Build history of the part. All positions in model axes, mm. Face numbers are marked on the shaded views. A direction names the side the tool comes from. Give positions to 0.01 mm unless a question says otherwise; leave off trailing zeros. Order: outer loops, then holes, each group sorted by start corner. A loop starts at its lowest first (then second) coordinate and runs counter-clockwise, first axis right, second up. Notation, with made-up numbers: (-19, 82.25) - (1, 82.25) arc R20 ccw to (1, 120.25) - close; hole circle Ø6 at (19, 32.25). An arc over 180 degrees is marked (long way). Use a Markdown table: item, result. Add a question column.
(1) Wall check: line 1 (X direction, y = 16.5, z = 31.5); line 2 (Y direction, x = -39, z = 24); line 3 (Z direction, x = -36, y = 10). Give the ranges that are in metal, low to high.
(2) Slice it at B-B (z = 19). Write the cut outline in (x, y), then the cut area to 3 significant figures.
(3) Slice it at A-A (x = -2). Write the cut outline in (y, z), then the cut area to 3 significant figures.
(4) Flat gauge pin, fed straight in: pin 1 (4 mm diameter, centred on x = 17.5, y = 17, fed in from -Z). Where does the tip first touch, or does it go through?
(5) Which spindle directions (+Z, -Z, +X, -X, +Y, -Y) get a long thin tool onto all of the face, cutting with end or side? Do the marked faces 1 and 2. Say none if no direction does.
(6) Slice it at C-C (y = 8). Write the cut outline in (x, z), then the cut area to 3 significant figures.
(7) Mould opens along Y. For the marked faces 3, 4 and 5 say: +Y half, -Y half, draft (parallel to the pull), parting line (faces both ways), or undercut.
from build123d import *

# Parameters (mm, degrees)
SKETCH_W        = 101
SKETCH_H        = 61
PAD_DEPTH       = 42.7
SKETCH001_W     = 91
SKETCH001_H     = 51
POCKET_DEPTH    = 32.7
CHAMFER_SIZE    = 2
CHAMFER001_SIZE = 2
CHAMFER002_SIZE = 2
CHAMFER003_SIZE = 2


with BuildPart() as part:
    # Sketch → Pad (new body)
    with BuildSketch(Plane.XY):
        Rectangle(SKETCH_W, SKETCH_H)
    extrude(amount=PAD_DEPTH)

    # Sketch001 (on Face5 of Pad) → Pocket (cut)
    with BuildSketch(Plane(origin=(0, 0, 0), x_dir=(1, 0, 0), z_dir=(0, 0, -1))):
        Rectangle(SKETCH001_W, SKETCH001_H)
    extrude(amount=-POCKET_DEPTH, mode=Mode.SUBTRACT)

    # Chamfer
    chamfer_edges = [part.edges().sort_by_distance(p)[0] for p in [
        (-50.5, -30.5, 21.35),
    ]]
    chamfer(chamfer_edges, length=CHAMFER_SIZE)

    # Chamfer001
    chamfer001_edges = [part.edges().sort_by_distance(p)[0] for p in [
        (-50.5, 30.5, 21.35),
    ]]
    chamfer(chamfer001_edges, length=CHAMFER001_SIZE)

    # Chamfer002
    chamfer002_edges = [part.edges().sort_by_distance(p)[0] for p in [
        (50.5, 30.5, 21.35),
        (50.5, -30.5, 21.35),
    ]]
    chamfer(chamfer002_edges, length=CHAMFER002_SIZE)

    # Chamfer003
    chamfer003_edges = [part.edges().sort_by_distance(p)[0] for p in [
        (0, 30.5, 42.7),
        (49.5, 29.5, 42.7),
        (-49.5, 29.5, 42.7),
        (50.5, 0, 42.7),
        (-50.5, 0, 42.7),
        (49.5, -29.5, 42.7),
        (-49.5, -29.5, 42.7),
        (0, -30.5, 42.7),
    ]]
    chamfer(chamfer003_edges, length=CHAMFER003_SIZE)


solid = part.part
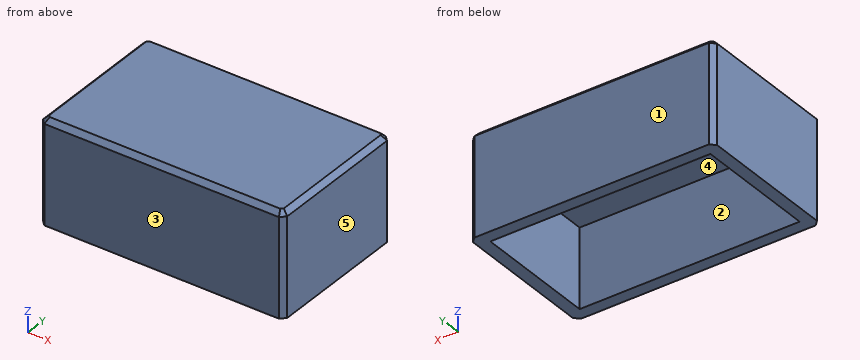
Solution:
| question | item | result |
|---|---|---|
| 1 | line 1 | -50.5 to -45.5, 45.5 to 50.5 |
| 1 | line 2 | -30.5 to -25.5, 25.5 to 30.5 |
| 1 | line 3 | 32.7 to 42.7 |
| 2 | outline | (-50.5, -28.5) - (-48.5, -30.5) - (48.5, -30.5) - (50.5, -28.5) - (50.5, 28.5) - (48.5, 30.5) - (-48.5, 30.5) - (-50.5, 28.5) - close; hole (-45.5, -25.5) - (45.5, -25.5) - (45.5, 25.5) - (-45.5, 25.5) - close |
| 2 | area | 1,510 mm2 |
| 3 | outline | (-30.5, 0) - (-25.5, 0) - (-25.5, 32.7) - (25.5, 32.7) - (25.5, 0) - (30.5, 0) - (30.5, 40.7) - (28.5, 42.7) - (-28.5, 42.7) - (-30.5, 40.7) - close |
| 3 | area | 933 mm2 |
| 4 | pin 1 | z = 32.7 |
| 5 | face 1 | +Z, -Z, +X, -X, +Y |
| 5 | face 2 | -Z |
| 6 | outline | (-50.5, 0) - (-45.5, 0) - (-45.5, 32.7) - (45.5, 32.7) - (45.5, 0) - (50.5, 0) - (50.5, 40.7) - (48.5, 42.7) - (-48.5, 42.7) - (-50.5, 40.7) - close |
| 6 | area | 1,330 mm2 |
| 7 | face 3 | -Y half |
| 7 | face 4 | undercut |
| 7 | face 5 | draft |
